```python
from build123d import *

# Parameters (mm, degrees)
F2_T = -8


with BuildPart() as f1:
    # F0 (on Front) → F1 (revolve)
    with BuildSketch(Plane.XZ):
        Polygon((0, 150), (0, 0), (40, 0), (40, 51.2300857674), (25.6093478629, 71.2300857674), (25.6093478629, 101.2300857674), (40, 106.2300857674), (40, 128), (25.6093478629, 138), (25.6093478629, 150), align=None)
    revolve(axis=Axis((0, 0, 75), (0, 0, -1)))

    # F2
    f2_openings = [f1.faces().sort_by_distance(p)[0] for p in [
        (0, 0, 150),
    ]]
    offset(amount=F2_T, openings=f2_openings, kind=Kind.INTERSECTION)


solid = f1.part
```
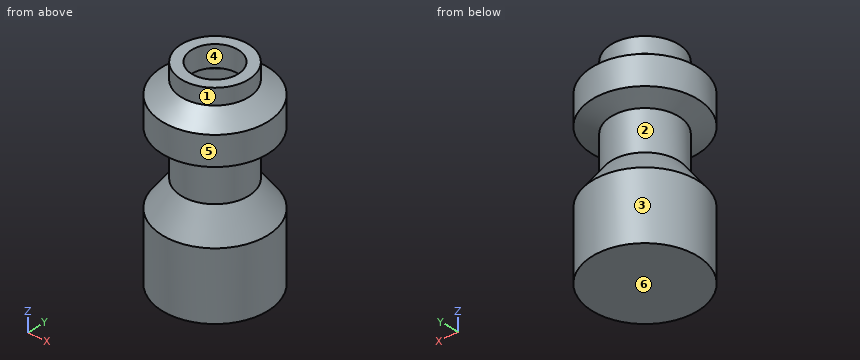
Source: CAD feature listing. Evaluate the final solid. Frame: model axes, mm. Face numbers are marked on the shaded views. A direction names the side the tool comes from. Round coordinates to 2 decimals unless told otherwise and drop trailing zeros. Order: outer loops, then holes, each group sorted by start corner. A loop starts at its lowest first (then second) coordinate and runs counter-clockwise, first axis right, second up. Notation, with made-up numbers: (-25.75, 65.25) -> (3.25, 65.25) arc R25 cw to (3.25, 86.25) -> close; hole circle Ø11 at (-34.75, 76.5). An arc over 180 degrees is marked (long way). One line per item, written item: value. Start each with the question number.
Q1. Material intervals for probe 1 along Y at (x, z) = (0, 38); probe 2 along Y at (x, z) = (0, 141); probe 3 along X at (y, z) = (6, 137.5), sorted ascending.
Q2. Section query C-C (z = 79). Return the cut outline in (x, y), plus the area to 3 significant figures.
Q3. Access query for the marked faces 1, 2 and 3. Directions: +Z, -Z, +X, -X, +Y, -Y. A direction counts if a zero-diameter tool reaches every point of the face in a straight line with its end or side. Return the directions, or none.
Q4. Section query D-D (x = -23). Give the number of separate pieces and of enclosed holes in the cut face, plus the area to 3 significant figures.
Q5. Draft query along X for the marked faces 4, 5 and 6. Return one class per face: pulls with the +X half, pulls with the -X half, needs draft (parallel to the pull), parting line crosses it, or undercut.
Q6. Pin query (flat end, axial travel): pin 1 (4 mm diameter, centred on x = 10.5, z = 55, fed in from -Y); pin 2 (1.5 mm diameter, centred on x = -28.5, z = 47, fed in from +Y); pin 3 (3 mm diameter, centred on y = 10, z = 23.5, fed in from +X); pin 4 (8 mm diameter, centred on x = -19, y = 20, fed in from +Z). Return the tip coordinate at first contact, or that it passes through.
Findings below:
1. probe 1: -40 to -32, 32 to 40
1. probe 2: -25.61 to -17.61, 17.61 to 25.61
1. probe 3: -25.64 to -16.56, 16.56 to 25.64
2. outline: circle Ø51.22 at (0, 0); hole circle Ø35.22 at (0, 0)
2. area: 1,090 mm²
3. face 1: +Z
3. face 2: none
3. face 3: +Z, -Z
4. separate pieces: 1
4. enclosed holes: 2
4. area: 4,370 mm²
5. face 4: undercut
5. face 5: parting line crosses it
5. face 6: needs draft
6. pin 1: y = -37.37
6. pin 2: y = 28.81
6. pin 3: x = 39.09
6. pin 4: z = 150
